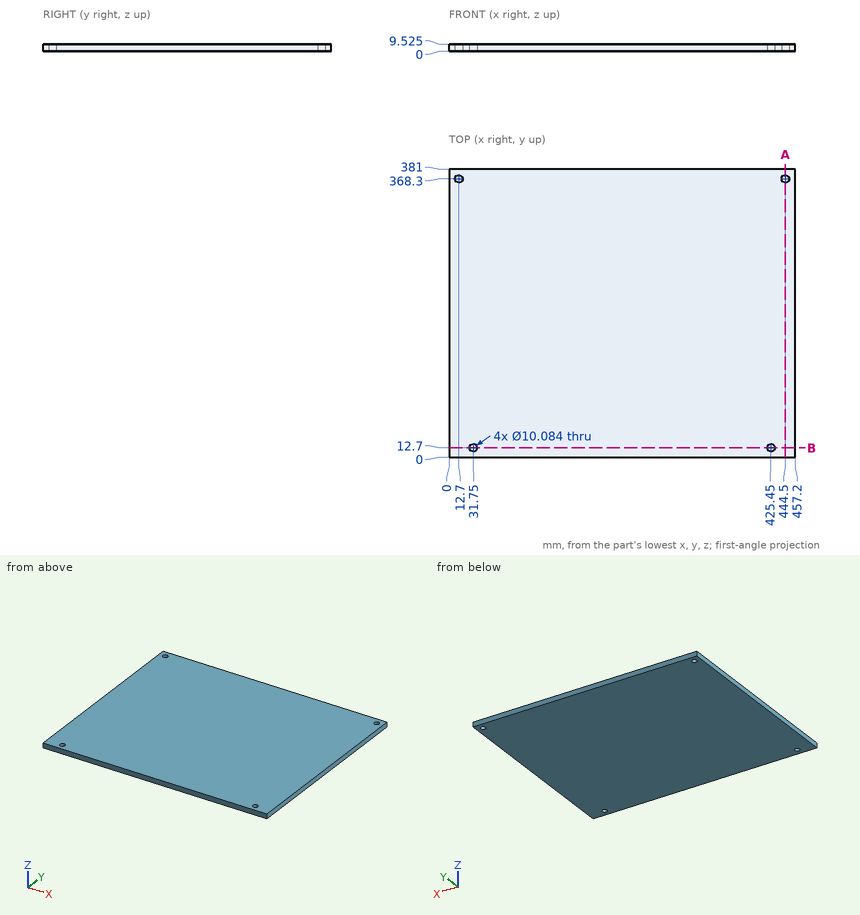
Source: three-view drawing plus pictorial views. Frame: mm from the lowest corner of the part. Give positions to 0.01 mm unless a question says otherwise; leave off trailing zeros. Write each loop counter-clockwise with the first axis right and the second up, starting at its lowest first coordinate (ties: lowest second). Pieces come first, ordered by that corner, then holes. Notation, with made-up numbers: (58.5, 63.5) - (68.5, 63.5) arc R23 cw to (68.5, 82.5) - close; hole circle Ø10 at (51, -26.5). An arc over 180 degrees is marked (long way). Write item = value, one per line. Start each with the question number.
Q1. Cut plane A-A, the plane x = 444.5. Return loops of the section in (y, z) (1 decimal).
Q2. Cut plane B-B, the plane y = 12.7. Return loops of the section in (x, z) (1 decimal), then the cut area to 3 significant figures.
Q3. Material intervals for probe 1 along X at (y, z) = (368.3, 6.75); probe 2 along Y at (x, z) = (425.45, 3); probe 3 along Y at (x, z) = (444.5, 3), sorted ascending.
Q4. Pin query (flat end, axial travel): pin 1 Ø8 at (x, y) = (425.45, 12.7) entering from -Z. Return the tip coordinate at first contact, or that it passes through.
Computed values:
q1.outline = (0, 0) - (363.3, 0) - (363.3, 9.5) - (0, 9.5) - close; (373.3, 0) - (381, 0) - (381, 9.5) - (373.3, 9.5) - close
q2.outline = (0, 0) - (26.7, 0) - (26.7, 9.5) - (0, 9.5) - close; (36.8, 0) - (420.4, 0) - (420.4, 9.5) - (36.8, 9.5) - close; (430.5, 0) - (457.2, 0) - (457.2, 9.5) - (430.5, 9.5) - close
q2.area = 4,160 mm²
q3.probe_1 = 0 to 7.66, 17.74 to 439.46, 449.54 to 457.2
q3.probe_2 = 0 to 7.66, 17.74 to 381
q3.probe_3 = 0 to 363.26, 373.34 to 381
q4.pin_1 = through
